The listing builds one solid part. Answer for the finished solid, in the listing's coordinates (mm). A direction names the side the tool comes from. Coordinates: 2 decimals unless noted, no trailing zeros. Loops run counter-clockwise (first coordinate to the right, second up) from the corner with the lowest first, then second, coordinate; pieces in that order, holes last. Notation, with made-up numbers: M 6.25,47.5 L 53.25,47.5 A23 ccw 53.25,70.5 Z; hole C 7,-11.75 d5. An arc over 180 degrees is marked long. Answer as a JSON object with one key per item and string values. Group by question number.
1. A cutting plane is placed at C-C on y = -20. Give the vertices of the cut face in (x, z), and give its area (3 significant figures).
2. For faces 4 (the face through (-47, 20.123, 6)), 5 (the face through (-40, 3.253, 18)), 6 (the face through (-47, -21.087, 6)), 7 (the face through (-47, 4, 12.7)), determine the directions among +Z, -Z, +X, -X, +Y, -Y from which every point of the face is accessible in a straight line to the end or side of a thin tool.
3. A cutting plane is placed at D-D on y = -5.5. Give the vertices of the cut face in (x, z), and give its area (3 significant figures).
4. Determine the mould class of faces 1 (the face through (-38, -0.681, 16)), 2 (the face through (-18.455, -14.151, 12.522)), 3 (the face through (-70.973, 0, 6)) for opening direction X: released by +X, released by -X, zero draft, split by the parting line, or undercut.
5. Straight lines are drawn through the part: L1, parallel to X at y = 0.5, z = 7.25; L2, parallel to Z at x = -50.5, y = 9; L3, parallel to Y at x = -18, z = 7. For each, find the intervals that lie inside material, in ascending order.
6. A cutting plane is placed at B-B on z = 5.25. Give the vertices of the cut face in (x, y).
7. Given pin 1 (2 mm diameter, centred on y = 16, z = 18, fed in from +X); pin 2 (12 mm diameter, centred on x = -33.5, y = -14, fed in from -Z); pin 3 (3 mm diameter, centred on y = -15.5, z = 19, fed in from -X); pin 4 (10 mm diameter, centred on x = -48.5, z = 4, fed in from +Y), each flat-ended and moving along its own axis, determine where each tip first touches the part or whether it passes through.
8. A cutting plane is placed at A-A on x = 0. Give the vertices of the cut face in (y, z).
from build123d import *

# Parameters (mm, degrees)
F0_R     = 23.255918
F1_DEPTH = 25.4
F2_DEPTH = 12.7
F4_DEPTH = 12.7
F6_DEPTH = 25.4


with BuildPart() as f1:
    # F0 (on Top) → F1 (new body)
    with BuildSketch(Plane.XY):
        with BuildLine():
            ThreePointArc((30.753419, 0), (10.737173, 28.818152), (-23.255918, 20.122997))
            ThreePointArc((-23.255918, 20.122997), (-30.745882, -0.680806), (-22.342394, -21.13268))
            ThreePointArc((-22.342394, -21.13268), (11.372505, -28.573395), (30.753419, 0))
        make_face()
        Circle(F0_R, mode=Mode.SUBTRACT)
    extrude(amount=F1_DEPTH)

    # F0 (on Top) → F2 (join)
    with BuildSketch(Plane.XY):
        with BuildLine():
            Line((-23.255918, 20.122997), (-70.972726, 20.122997))
            Line((-70.972726, 20.122997), (-70.972726, -21.086972))
            Line((-70.972726, -21.086972), (-23.255918, -21.086972))
            Line((-23.255918, -21.086972), (-22.342394, -21.13268))
            ThreePointArc((-22.342394, -21.13268), (-30.745882, -0.680806), (-23.255918, 20.122997))
        make_face()
    extrude(amount=F2_DEPTH)

    # F3 (on face) → F4 (join)
    with BuildSketch(Plane.XY.offset(12.7)):
        with BuildLine():
            ThreePointArc((-30.745882, -0.680806), (-30.726394, 1.288977), (-30.580838, 3.253472))
            Line((-30.580838, 3.253472), (-55.966172, 3.253472))
            Line((-55.966172, 3.253472), (-55.966172, -0.680806))
            Line((-55.966172, -0.680806), (-30.745882, -0.680806))
        make_face()
    extrude(amount=F4_DEPTH)

    # F5 (on face) → F6 (cut)
    with BuildSketch(Plane(origin=(0, 3.253472, 0), x_dir=(-1, 0, 0), z_dir=(0, 1, 0))):
        Polygon((55.966172, 25.4), (30.580838, 25.4), (55.966172, 12.7), align=None)
    extrude(amount=-F6_DEPTH, mode=Mode.SUBTRACT)


solid = f1.part
From the geometry:
{
 "1": {"outline": "M -70.97,0 L -11.87,0 L -11.87,25.4 L -23.36,25.4 L -23.36,12.7 L -70.97,12.7 Z; M 11.87,0 L 23.36,0 L 23.36,25.4 L 11.87,25.4 Z", "area": "1,190 mm²"},
 "2": {"face 4": "+Z, -Z, -X, +Y", "face 5": "+Z, -X, +Y", "face 6": "+Z, -Z, -X, -Y", "face 7": "+Z, -X"},
 "3": {"outline": "M -70.97,0 L -22.6,0 L -22.6,25.4 L -30.26,25.4 L -30.26,12.7 L -70.97,12.7 Z; M 22.6,0 L 30.26,0 L 30.26,25.4 L 22.6,25.4 Z", "area": "906 mm²"},
 "4": {"face 1": "zero draft", "face 2": "undercut", "face 3": "released by -X"},
 "5": {"L1": "x = -70.97 to -23.25, 23.25 to 30.75", "L2": "z = 0 to 12.7", "L3": "y = -24.94 to -14.73, 14.73 to 24.94"},
 "6": {"outline": "M -70.97,-21.09 L -23.26,-21.09 L -22.34,-21.13 A30.75 ccw long -23.26,20.12 L -70.97,20.12 Z; hole C 0,0 d46.51"},
 "7": {"pin 1": "stops at x = 26.85", "pin 2": "stops at z = 0", "pin 3": "stops at x = -27.38", "pin 4": "stops at y = 20.12"},
 "8": {"outline": "M -30.75,0 L -23.26,0 L -23.26,25.4 L -30.75,25.4 Z; M 23.26,0 L 30.75,0 L 30.75,25.4 L 23.26,25.4 Z"}
}
